Geometry: final body of the model. Coordinates: model frame, mm. Face numbers are marked on the shaded views. A direction names the side the tool comes from. Give positions to 0.01 mm unless a question says otherwise; leave off trailing zeros. Write each loop counter-clockwise with the first axis right and the second up, starting at its lowest first coordinate (ties: lowest second). Pieces come first, ordered by that corner, then holes. Notation, with made-up numbers: (-10, -16) -> (12, -16) arc R30 ccw to (12, 12) -> close; hole circle Ø8 at (3.25, 10.5). An arc over 180 degrees is marked (long way). Answer as a JSON object with one key per item and string values.
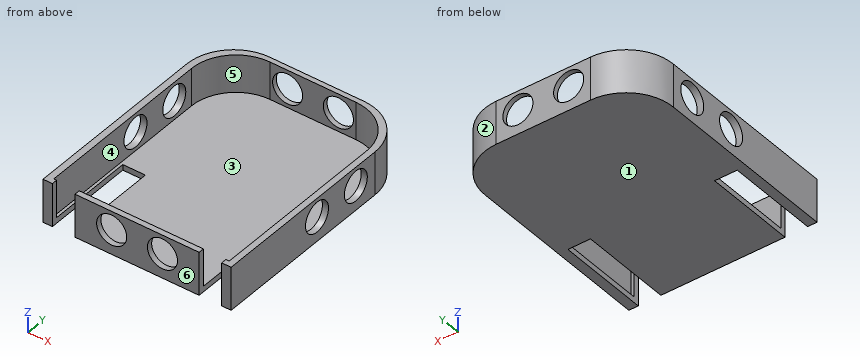
from build123d import *

# Parameters (mm, degrees)
PAD_DEPTH       = 23
POCKET_DEPTH    = 20
SKETCH002_R     = 8
POCKET001_DEPTH = 100.001
SKETCH003_R     = 8
POCKET002_DEPTH = 125.001
SKETCH004_W     = 12
SKETCH004_H     = 50
POCKET003_DEPTH = 23.001


with BuildPart() as part:
    # Sketch → Pad (new body)
    with BuildSketch(Plane.XY):
        with BuildLine():
            Line((-50, 38.45712), (-50, -61.54288))
            Line((-50, -61.54288), (50, -61.54288))
            Line((50, -61.54288), (50, 38.45712))
            ThreePointArc((50, 38.45712), (42.67767, 56.13479), (25, 63.45712))
            Line((25, 63.45712), (-25, 63.45712))
            ThreePointArc((-25, 63.45712), (-42.67767, 56.13479), (-50, 38.45712))
        make_face()
    extrude(amount=PAD_DEPTH)

    # Sketch001 → Pocket (cut)
    with BuildSketch(Plane.XY.offset(23)):
        with BuildLine():
            Line((-46.504223, 37.299377), (-46.504223, -58.589802))
            Line((-46.504223, -58.589802), (46.756358, -58.589802))
            Line((46.756358, -58.589802), (46.756358, 36.931984))
            ThreePointArc((46.756358, 36.931984), (39.747359, 53.853203), (22.82614, 60.862202))
            Line((22.82614, 60.862202), (-22.941398, 60.862202))
            ThreePointArc((-22.941398, 60.862202), (-39.602831, 53.96081), (-46.504223, 37.299377))
        make_face()
    extrude(amount=-POCKET_DEPTH, mode=Mode.SUBTRACT)

    # Sketch002 → Pocket001 (cut, through all)
    with BuildSketch(Plane.YZ.offset(50)):
        with Locations((-1.771652, 13)):
            Circle(SKETCH002_R)
        with Locations((25.228348, 13)):
            Circle(SKETCH002_R)
    extrude(amount=-POCKET001_DEPTH, mode=Mode.SUBTRACT)

    # Sketch003 → Pocket002 (cut, through all)
    with BuildSketch(Plane.XZ.offset(61.54288)):
        with Locations((-13.5, 13)):
            Circle(SKETCH003_R)
        with Locations((13.5, 13)):
            Circle(SKETCH003_R)
    extrude(amount=-POCKET002_DEPTH, mode=Mode.SUBTRACT)

    # Sketch004 → Pocket003 (cut, through all)
    with BuildSketch(Plane(origin=(0, 0, 0), x_dir=(1, 0, 0), z_dir=(0, 0, -1))):
        with Locations((-39, 37.553897)):
            Rectangle(SKETCH004_W, SKETCH004_H)
        with Locations((39, 37.553897)):
            Rectangle(SKETCH004_W, SKETCH004_H)
    extrude(amount=-POCKET003_DEPTH, mode=Mode.SUBTRACT)


solid = part.part
Q1. Cut plane D-D (y = 14.5). Return the cut outline in (x, z), and give its area (3 significant figures).
Values:
{"outline": "(-50, 0) -> (50, 0) -> (50, 23) -> (46.76, 23) -> (46.76, 3) -> (-46.5, 3) -> (-46.5, 23) -> (-50, 23) -> close", "area": "435 mm²"}
Q2. Cut plane B-B (x = 13.5). Return the cut outline in (y, z).
Values:
{"outline": "(-61.54, 0) -> (63.46, 0) -> (63.46, 5) -> (60.86, 5) -> (60.86, 3) -> (-58.59, 3) -> (-58.59, 5) -> (-61.54, 5) -> close; (-61.54, 21) -> (-58.59, 21) -> (-58.59, 23) -> (-61.54, 23) -> close; (60.86, 21) -> (63.46, 21) -> (63.46, 23) -> (60.86, 23) -> close"}
Q3. Set-up query: the marked faces 5 and 6. Return all of +Z, -Z, +X, -X, +Y, -Y with unobstructed straight access to the full face (end or side cutting, diameter ignored); none if empty.
Values:
{"face 5": "+Z", "face 6": "+Z, -Z, +X, -X, -Y"}
Q4. Mould query, pull axis X, two halves, no side actions, for the marked faces 1, 2, 3 and 4. Classes: pulls with the +X half, pulls with the -X half, needs draft (parallel to the pull), parting line crosses it, or undercut.
Values:
{"face 1": "needs draft", "face 2": "pulls with the +X half", "face 3": "undercut", "face 4": "undercut"}
Q5. Material intervals for L1, parallel to X at y = -44.5, z = 11; L2, parallel to Y at x = -6.5, z = 18.75; L3, parallel to Z at x = 13, y = -59, sorted ascending. Write a range as from..to.
Values:
{"L1": "-50..-46.5, 46.76..50", "L2": "-61.54..-58.59, 60.86..63.46", "L3": "0..5.02, 20.98..23"}
Q6. First-contact query: P1, Ø3, axis at x = -27, z = 12.5, coming from the +Y side; P2, Ø1, axis at x = 20.5, y = 40.5, coming from the +Z side; P3, Ø0.9, axis at x = 46, z = 12, coming from the +Y side. Flat tips, straight axial feed; report the tip coordinate or a pass-through.
Values:
{"P1": "y = 63.45", "P2": "z = 3", "P3": "y = 52.69"}
Q7. Cut plane A-A (y = -22). Return the cut outline in (x, z), and give its area (3 significant figures).
Values:
{"outline": "(-50, 0) -> (-45, 0) -> (-45, 3) -> (-46.5, 3) -> (-46.5, 23) -> (-50, 23) -> close; (-33, 0) -> (33, 0) -> (33, 3) -> (-33, 3) -> close; (45, 0) -> (50, 0) -> (50, 23) -> (46.76, 23) -> (46.76, 3) -> (45, 3) -> close", "area": "363 mm²"}
Q8. Cut plane C-C (x = 3). Return the cut outline in (y, z), and give its area (3 significant figures).
Values:
{"outline": "(-61.54, 0) -> (63.46, 0) -> (63.46, 23) -> (60.86, 23) -> (60.86, 3) -> (-58.59, 3) -> (-58.59, 23) -> (-61.54, 23) -> close", "area": "486 mm²"}
